```python
from build123d import *

# Parameters (mm, degrees)
SKETCH_3_W               = 6.02
SKETCH_3_H               = 6.2
EXTRUDE_1_DEPTH          = 3
SKETCH_4_W               = 1.5
SKETCH_4_H               = 4
CUT_EXTRUDE_1_DEPTH      = 0.5
CUT_EXTRUDE_2_DEPTH      = 8.406105589
SKETCH_6_W               = 0.5
SKETCH_6_H               = 0.25
PATTERN_LINEAR_1_COUNT   = 2
PATTERN_LINEAR_1_PITCH   = 2.54
MIRROR_1_COPY_1_SKETCH_W = 0.5
MIRROR_1_COPY_1_SKETCH_H = 0.25


with BuildPart() as part:
    # Эскиз3 → Бобышка-Вытянуть1 (new body)
    with BuildSketch(Plane(origin=(0, 0, 0), x_dir=(1, 0, 0), z_dir=(0, 1, 0))):
        Rectangle(SKETCH_3_W, SKETCH_3_H)
    extrude(amount=EXTRUDE_1_DEPTH)

    # Эскиз4 → Вырез-Вытянуть1 (cut)
    with BuildSketch(Plane(origin=(0, 3, 0), x_dir=(1, 0, 0), z_dir=(0, 1, 0))):
        with Locations((-1.253333333, 0)):
            Rectangle(SKETCH_4_W, SKETCH_4_H)
        with Locations((1.253333333, 0)):
            Rectangle(SKETCH_4_W, SKETCH_4_H)
    extrude(amount=-CUT_EXTRUDE_1_DEPTH, mode=Mode.SUBTRACT)

    # Эскиз5 → Вырез-Вытянуть2 (cut, through all)
    with BuildSketch(Plane(origin=(3.01, 0, 0), x_dir=(0, 0, -1), z_dir=(1, 0, 0))):
        Polygon((-3.1, 0.95), (-2.8, 0), (-3.1, 0), align=None)
        Polygon((3.1, 0), (2.8, 0), (3.1, 0.95), align=None)
    extrude(amount=-CUT_EXTRUDE_2_DEPTH, mode=Mode.SUBTRACT)

    # По траектории1: sweep along a curve in space
    with BuildLine() as sweep_1_path:
        Line((-1.27, 1.075, 3.1), (-1.27, 1.075, 3.41))
        ThreePointArc((-1.27, 1.075, 3.41), (-1.27, 0.957842712, 3.692842712), (-1.27, 0.675, 3.81))
        Line((-1.27, 0.675, 3.81), (-1.27, -0.15, 3.81))
        ThreePointArc((-1.27, -0.15, 3.81), (-1.27, -0.645, 3.315), (-1.27, -0.15, 2.82))
    # Эскиз6 → По траектории1 (sweep)
    with BuildSketch(Plane.XY.offset(3.1)):
        with Locations((-1.27, 1.075)):
            Rectangle(SKETCH_6_W, SKETCH_6_H)
    sweep_1 = sweep(path=sweep_1_path.line)

    # Линейный массив1: По траектории1 ×2
    with Locations(*[(i * PATTERN_LINEAR_1_PITCH, 0, 0) for i in range(1, PATTERN_LINEAR_1_COUNT)]):
        add(sweep_1)

    # Зеркальное отражение1: По траектории1 across plane
    add(sweep_1.mirror(Plane.XY))

    # Зеркальное отражение1 copy 1: sweep along a curve in space
    with BuildLine() as mirror_1_copy_1_path:
        Line((1.27, 1.075, -3.1), (1.27, 1.075, -3.41))
        ThreePointArc((1.27, 1.075, -3.41), (1.27, 0.957842712, -3.692842712), (1.27, 0.675, -3.81))
        Line((1.27, 0.675, -3.81), (1.27, -0.15, -3.81))
        ThreePointArc((1.27, -0.15, -3.81), (1.27, -0.645, -3.315), (1.27, -0.15, -2.82))
    # Зеркальное отражение1 copy 1 sketch → Зеркальное отражение1 copy 1 (sweep)
    with BuildSketch(Plane(origin=(2.54, 0, -3.1), x_dir=(1, 0, 0), z_dir=(0, 0, -1))):
        with Locations((-1.27, -1.075)):
            Rectangle(MIRROR_1_COPY_1_SKETCH_W, MIRROR_1_COPY_1_SKETCH_H)
    sweep(path=mirror_1_copy_1_path.line)


solid = part.part
```
For this review, take the finished solid that the model builds, in its own axes (mm). A direction names the side the tool comes from. Round coordinates to 2 decimals unless told otherwise and drop trailing zeros. Order: outer loops, then holes, each group sorted by start corner. A loop starts at its lowest first (then second) coordinate and runs counter-clockwise, first axis right, second up. Notation, with made-up numbers: (26, -39) -> (30, -39) arc R31 ccw to (30, -1) -> close; hole circle Ø9 at (3.5, -14). An arc over 180 degrees is marked (long way). Use a Markdown table: item, result.
Item 1: Machinability: for faces 1 (the flat face through (0.04, 0.48, 2.95)), 2 (the flat face through (1, 2.5, 0)), 3 (the flat face through (0, 3, 0)), which of the approach directions +Z, -Z, +X, -X, +Y, -Y give a long, thin tool a straight path to every point of the face, cutting with its end or side? Answer none if there is none.
Resolved:
| item | result |
|---|---|
| face 1 | +X, -X |
| face 2 | +Y |
| face 3 | +Z, -Z, +X, -X, +Y |
Item 2: Take a section at B-B (x = 0). State the section outline as (y, z) points.
Resolved:
| item | result |
|---|---|
| outline | (0, -2.8) -> (0.95, -3.1) -> (3, -3.1) -> (3, 3.1) -> (0.95, 3.1) -> (0, 2.8) -> close |
Item 3: Take a section at A-A (z = -1). State the section outline as (x, y) points, plus the area to 3 significant figures.
Resolved:
| item | result |
|---|---|
| outline | (-3.01, 0) -> (3.01, 0) -> (3.01, 3) -> (2, 3) -> (2, 2.5) -> (0.5, 2.5) -> (0.5, 3) -> (-0.5, 3) -> (-0.5, 2.5) -> (-2, 2.5) -> (-2, 3) -> (-3.01, 3) -> close |
| area | 16.6 mm² |
Item 4: Draft analysis for pull direction X (two halves, no side actions). For faces 4 (the flat face through (0, 0, 0)), 5 (the flat face through (-1, 2.5, 0)), 6 (the flat face through (-3.01, 1, 0)), state which applies: +X half, -X half, draft (parallel to the pull), parting line (faces both ways), or undercut.
Resolved:
| item | result |
|---|---|
| face 4 | draft |
| face 5 | undercut |
| face 6 | -X half |
Item 5: For line 1 along X through (y, z) = (2.55, -1); line 2 along Y through (x, z) = (-0.25, -2.5); line 3 along Y through (x, z) = (-1.25, 1.25), list the stretches that pass through material, from the lowest coordinate up. Write a range as [from, to].
Resolved:
| item | result |
|---|---|
| line 1 | x = [-3.01, -2], [-0.5, 0.5], [2, 3.01] |
| line 2 | y = [0, 3] |
| line 3 | y = [0, 2.5] |
Item 6: For pin 1 (1 mm diameter, centred on x = 0.5, y = 2, fed in from -Z); pin 2 (0.8 mm diameter, centred on x = -1, z = 0.5, fed in from +Y); pin 3 (3 mm diameter, centred on x = -1, z = 1.5, fed in from -Y), all flat-tipped, find the tip position at first contact; note any pin that passes through.
Resolved:
| item | result |
|---|---|
| pin 1 | stops at z = -3.1 |
| pin 2 | stops at y = 2.5 |
| pin 3 | stops at y = -0.68 |
